For this review, take the finished solid that the model builds, in its own axes (mm). Round coordinates to 2 decimals unless told otherwise and drop trailing zeros. Order: outer loops, then holes, each group sorted by start corner. A loop starts at its lowest first (then second) coordinate and runs counter-clockwise, first axis right, second up. Notation, with made-up numbers: (45.25, 65) -> (92.25, 65) arc R20 ccw to (92.25, 85) -> close; hole circle Ø7 at (-10, 0.25). An arc over 180 degrees is marked (long way). Use a Markdown table: item, result. Add a question column.
1) Consider section B-B (x = 0). State the section outline as (y, z) points, plus the area to 3 significant figures.
2) Clearance check with a flat-ended pin moving along its axis: P1, Ø1.9, axis at x = -15.5, z = -15.5, coming from the -Y side. State where the tip first meets the part, or that it passes through.
3) Consider section D-D (x = -15.5). State the section outline as (y, z) points.
4) Consider section C-C (z = 25.2). State the section outline as (x, y) points, plus the area to 3 significant figures.
5) Wall thickness on line 1 along Z through (x, y) = (27, 5.15); line 2 along Z through (x, y) = (15.5, 4.75); line 3 along X through (y, z) = (4.3, 25.2): over which ranges is each line inside the solid? List them lowest first. Write a range as [from, to].
6) Consider section A-A (y = 2.6). Give the number of separate pieces and of enclosed holes in the cut face, plus the area to 3 significant figures.
7) Draft analysis for pull direction X (two halves, no side actions). For faces 1 (the face through (0, 3, 30.2)), 2 (the face through (-31, 3, 5)), 3 (the face through (-13.9, 2.96, 15.43)), state which applies: pulls with the +X half, pulls with the -X half, needs draft (parallel to the pull), parting line crosses it, or undercut.
```python
from build123d import *

# Parameters (mm, degrees)
SKETCH1_W                  = 63
SKETCH1_H                  = 51.2
BOSS_EXTRUDE1_DEPTH        = 6
M5_CLEARANCE_HOLE1_D       = 5.3
M3_CLEARANCE_HOLE1_D       = 3.2
F_22_0_22_DIAMETER_HOLE1_D = 22


with BuildPart() as part:
    # Sketch1 → Boss-Extrude1 (new body)
    with BuildSketch(Plane(origin=(0, 0, 0), x_dir=(1, 0, 0), z_dir=(0, 1, 0))):
        with Locations((0.5, -4.6)):
            Rectangle(SKETCH1_W, SKETCH1_H)
    extrude(amount=BOSS_EXTRUDE1_DEPTH)

    # M5 Clearance Hole1 (through all)
    with Locations(Plane(origin=(0, 6, 0), x_dir=(1, 0, 0), z_dir=(0, 1, 0))):
        with Locations((-26, 16), (-26, -25.2), (27, -25.2), (27, 16)):
            Hole(M5_CLEARANCE_HOLE1_D / 2)

    # M3 Clearance Hole1 (through all)
    with Locations(Plane(origin=(0, 6, 0), x_dir=(1, 0, 0), z_dir=(0, 1, 0))):
        with Locations((-15.5, 15.5), (15.5, 15.5), (15.5, -15.5), (-15.5, -15.5)):
            Hole(M3_CLEARANCE_HOLE1_D / 2)

    # Ø22.0 (22) Diameter Hole1 (through all)
    with Locations(Plane(origin=(0, 6, 0), x_dir=(1, 0, 0), z_dir=(0, 1, 0))):
        with Locations((0, 0)):
            Hole(F_22_0_22_DIAMETER_HOLE1_D / 2)


solid = part.part
```
Results list:
| question | item | result |
|---|---|---|
| 1 | outline | (0, -21) -> (6, -21) -> (6, -11) -> (0, -11) -> close; (0, 11) -> (6, 11) -> (6, 30.2) -> (0, 30.2) -> close |
| 1 | area | 175 mm2 |
| 2 | P1 | through |
| 3 | outline | (0, -21) -> (6, -21) -> (6, -17.1) -> (0, -17.1) -> close; (0, -13.9) -> (6, -13.9) -> (6, 13.9) -> (0, 13.9) -> close; (0, 17.1) -> (6, 17.1) -> (6, 30.2) -> (0, 30.2) -> close |
| 4 | outline | (-31, 0) -> (-28.65, 0) -> (-28.65, 6) -> (-31, 6) -> close; (-23.35, 0) -> (24.35, 0) -> (24.35, 6) -> (-23.35, 6) -> close; (29.65, 0) -> (32, 0) -> (32, 6) -> (29.65, 6) -> close |
| 4 | area | 314 mm2 |
| 5 | line 1 | [-21, -18.65], [-13.35, 22.55], [27.85, 30.2] |
| 5 | line 2 | [-21, -17.1], [-13.9, 13.9], [17.1, 30.2] |
| 5 | line 3 | [-31, -28.65], [-23.35, 24.35], [29.65, 32] |
| 6 | separate pieces | 1 |
| 6 | enclosed holes | 9 |
| 6 | area | 2,730 mm2 |
| 7 | face 1 | needs draft |
| 7 | face 2 | pulls with the -X half |
| 7 | face 3 | undercut |
